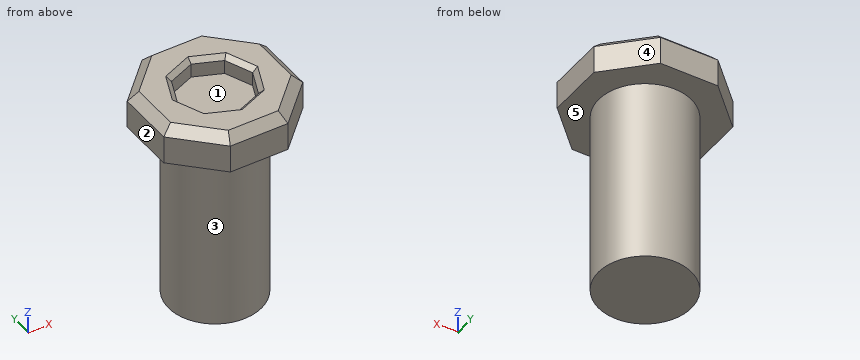
Solid Edge part; units mm, degrees
sketch "Sketch1" plane through (0, 0, 0) normal (0, 0, 1) x (1, 0, 0)
  line L0 (19.05, -7.8908) -> (19.05, 7.8908)
  line L1 (19.05, 7.8908) -> (7.8908, 19.05)
  line L2 (7.8908, 19.05) -> (-7.8908, 19.05)
  line L3 (-7.8908, 19.05) -> (-19.05, 7.8908)
  line L4 (-19.05, 7.8908) -> (-19.05, -7.8908)
  line L5 (-19.05, -7.8908) -> (-7.8908, -19.05)
  line L6 (-7.8908, -19.05) -> (7.8908, -19.05)
  line L7 (7.8908, -19.05) -> (19.05, -7.8908)
extrude "Protrusion1" add sketch "Sketch1" along normal blind 10.16
sketch "Sketch2" plane through (0, 0, 0) normal (0, 0, 1) x (1, 0, 0)
  circle A0 centre (0, 0) radius 12.7
extrude "ExtrudedProtrusion_2" add sketch "Sketch2" against normal blind 50.8
sketch "Sketch3" plane through (0, 0, 10.16) normal (0, 0, 1) x (0, 1, 0)
  line L0 (-10.3098, 0) -> (-7.2901, -7.2901)
  line L1 (-7.2901, -7.2901) -> (0, -10.3098)
  line L2 (0, -10.3098) -> (7.2901, -7.2901)
  line L3 (7.2901, -7.2901) -> (10.3098, 0)
  line L4 (10.3098, 0) -> (7.2901, 7.2901)
  line L5 (7.2901, 7.2901) -> (0, 10.3098)
  line L6 (0, 10.3098) -> (-7.2901, 7.2901)
  line L7 (-7.2901, 7.2901) -> (-10.3098, 0)
extrude "ExtrudedCutout_1" cut sketch "Sketch3" against normal blind 5.08
chamfer "Chamfer_1" distance 1.27 angle 45 8 edges at (-8.8, 3.6451, 10.16) (-3.6451, 8.8, 10.16) (3.6451, 8.8, 10.16) (8.8, 3.6451, 10.16) (8.8, -3.6451, 10.16) (3.6451, -8.8, 10.16) (-3.6451, -8.8, 10.16) (-8.8, -3.6451, 10.16)
chamfer "Chamfer_2" distance 2.54 angle 45 8 edges at (13.4704, -13.4704, 10.16) (19.05, 0, 10.16) (13.4704, 13.4704, 10.16) (0, 19.05, 10.16) (-13.4704, 13.4704, 10.16) (-19.05, 0, 10.16) (-13.4704, -13.4704, 10.16) (0, -19.05, 10.16)
Input: part model. Units: mm. Frame: model coordinates. Face numbers are marked on the shaded views. A direction names the side the tool comes from. Coordinates: 2 decimals unless noted, no trailing zeros. Write each loop counter-clockwise with the first axis right and the second up, starting at its lowest first coordinate (ties: lowest second). Pieces come first, ordered by that corner, then holes.
1) Material intervals for line 1 along Z through (x, y) = (-14.5, 3); line 2 along Z through (x, y) = (-3, 0.5); line 3 along X through (y, z) = (0.5, -35.5), sorted ascending.
2) Section C-C on x = 13.5. Output: boundary loops of the cut face in (y, z), and give its area (3 significant figures).
3) Mould query, pull axis Y, two halves, no side actions, for the marked faces 1, 2 and 3. Classes: pulls with the +Y half, pulls with the -Y half, needs draft (parallel to the pull), parting line crosses it, or undercut.
4) Section B-B on z = -33. Output: boundary loops of the cut face in (x, y), and give its area (3 significant figures).
5) Set-up query: the marked faces 4 and 5. Return all of +Z, -Z, +X, -X, +Y, -Y with unobstructed straight access to the full face (end or side cutting, diameter ignored); none if empty.
6) Pin query (flat end, axial travel): pin 1 Ø3 at (y, z) = (9.5, -44.5) entering from -X; pin 2 Ø5 at (y, z) = (-14, -16) entering from +X; pin 3 Ø12 at (x, z) = (9, -17.5) entering from -Y. Return the tip coordinate at first contact, or that it passes through.
7) Section A-A on y = 2. Output: boundary loops of the cut face in (x, z).
8) Section D-D on y = -6. Output: boundary loops of the cut face in (x, z).
Check result:
1. line 1: z = 0 to 10.16
1. line 2: z = -50.8 to 5.08
1. line 3: x = -12.69 to 12.69
2. outline: (-13.44, 0) - (13.44, 0) - (13.44, 7.62) - (9.85, 10.16) - (-9.85, 10.16) - (-13.44, 7.62) - close
2. area: 264 mm2
3. face 1: undercut
3. face 2: needs draft
3. face 3: parting line crosses it
4. outline: circle Ø25.4 at (0, 0)
4. area: 507 mm2
5. face 4: +Z, -Z, +X, +Y
5. face 5: -Z
6. pin 1: stops at x = -9.86
6. pin 2: stops at x = 5.39
6. pin 3: stops at y = -12.34
7. outline: (-19.05, 0) - (-12.54, 0) - (-12.54, -50.8) - (12.54, -50.8) - (12.54, 0) - (19.05, 0) - (19.05, 7.62) - (16.51, 10.16) - (10.86, 10.16) - (9.48, 8.89) - (9.48, 5.08) - (-9.48, 5.08) - (-9.48, 8.89) - (-10.86, 10.16) - (-16.51, 10.16) - (-19.05, 7.62) - close
8. outline: (-19.05, 0) - (-11.19, 0) - (-11.19, -50.8) - (11.19, -50.8) - (11.19, 0) - (19.05, 0) - (19.05, 7.62) - (16.51, 10.16) - (9.2, 10.16) - (7.82, 8.89) - (7.82, 5.08) - (-7.82, 5.08) - (-7.82, 8.89) - (-9.2, 10.16) - (-16.51, 10.16) - (-19.05, 7.62) - close
